Here's how the part is built. I have some questions about the finished solid (model axes, mm). Face numbers are marked on the shaded views. A direction names the side the tool comes from. Give positions to 0.01 mm unless a question says otherwise; leave off trailing zeros. Write each loop counter-clockwise with the first axis right and the second up, starting at its lowest first coordinate (ties: lowest second). Pieces come first, ordered by that corner, then holes. Notation, with made-up numbers: (-33, 26) - (-29, 26) arc R5 ccw to (-29, 31) - close; hole circle Ø7 at (19, -18.75). An arc over 180 degrees is marked (long way). One line per item, written item: value. Start each with the question number.
1) Imagine slicing it at C-C on y = 24.5. Write out the boundary of the cut face in (x, z).
2) Imagine slicing it at D-D on y = 66. Write out the boundary of the cut face in (x, z).
3) Imagine slicing it at A-A on x = -23. Write out the boundary of the cut face in (y, z), plus the area to 3 significant figures.
4) Imagine slicing it at B-B on z = 0. Write out the boundary of the cut face in (x, y) (3 decimals), plus the area to 3 significant figures.
5) We'd pull the mould along Y, two halves only. Please class the marked faces 1, 2, 3 and 4: +Y half, -Y half, draft (parallel to the pull), parting line (faces both ways), or undercut.
6) I'm going to push flat-ended pins straight in: P1, Ø6, axis at y = 13, z = 14.5, coming from the -X side; P2, Ø5, axis at x = -46.5, z = -15, coming from the -Y side; P3, Ø12, axis at y = 49, z = -1, coming from the -X side. Where does each tip first touch, or does it pass through?
7) On a 3-axis mill with a long thin cutter (end or side, diameter ignored), from which of +Z, -Z, +X, -X, +Y, -Y can I reach the whole of each face in a straight line? I mean the marked faces 5 and 6. Say none if no direction works.
8) Please list where these lines run through material, in increasing order: L1, parallel to Y at x = -27.5, z = 9; L2, parallel to X at y = 79, z = -14; L3, parallel to Y at x = -55.5, z = -8. Write a range as [from, to].
from build123d import *

# Parameters (mm, degrees)
EXTRUDE_THIN1_DEPTH = 19.05
SKETCH2_R           = 6.35
CUT_EXTRUDE1_DEPTH  = 10


with BuildPart() as part:
    # Sketch1 → Extrude-Thin1 (new, symmetric)
    with BuildSketch(Plane.XY):
        with BuildLine():
            Line((-77.216, 27.494), (-45.335245866, 0.74281114))
            ThreePointArc((-45.335245866, 0.74281114), (-44.380308124, 0.191476527), (-43.294392527, 0))
            Line((-43.294392527, 0), (-3.175, 0))
            ThreePointArc((-3.175, 0), (-0.92993597, 0.92993597), (0, 3.175))
            Line((0, 3.175), (0, 79.375))
            ThreePointArc((0, 79.375), (-0.92993597, 81.62006403), (-3.175, 82.55))
            Line((-3.175, 82.55), (-57.15, 82.55))
            Line((-57.15, 82.55), (-57.15, 88.9))
            Line((-57.15, 88.9), (-3.175, 88.9))
            ThreePointArc((-3.175, 88.9), (3.560192091, 86.110192091), (6.35, 79.375))
            Line((6.35, 79.375), (6.35, 3.175))
            ThreePointArc((6.35, 3.175), (3.560192091, -3.560192091), (-3.175, -6.35))
            Line((-3.175, -6.35), (-43.294392527, -6.35))
            ThreePointArc((-43.294392527, -6.35), (-46.55213932, -5.775570419), (-49.416952544, -4.121566579))
            Line((-49.416952544, -4.121566579), (-81.297706678, 22.629622281))
            Line((-81.297706678, 22.629622281), (-77.216, 27.494))
        make_face()
    extrude(amount=EXTRUDE_THIN1_DEPTH, both=True)

    # Sketch2 → Cut-Extrude1 (cut)
    with BuildSketch(Plane(origin=(0, 88.9, 0), x_dir=(1, 0, 0), z_dir=(0, 1, 0))):
        with Locations(Location((-44.45, 0, 0), (0, 0, 270))):
            Circle(SKETCH2_R)
    extrude(amount=-CUT_EXTRUDE1_DEPTH, mode=Mode.SUBTRACT)


solid = part.part
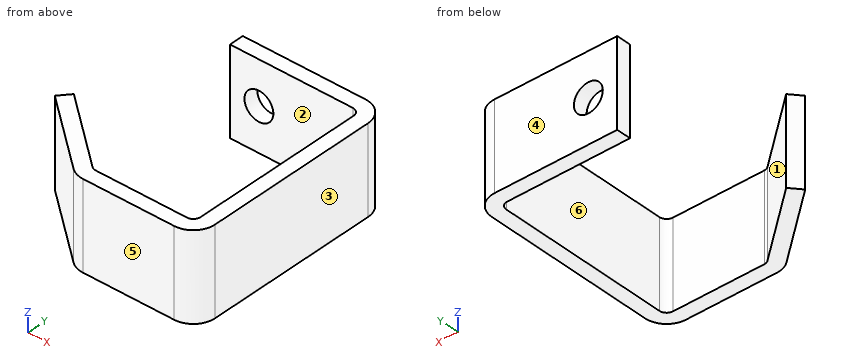
Numbers:
1. outline: (-79.73, -19.05) - (-73.65, -19.05) - (-73.65, 19.05) - (-79.73, 19.05) - close; (0, -19.05) - (6.35, -19.05) - (6.35, 19.05) - (0, 19.05) - close
2. outline: (0, -19.05) - (6.35, -19.05) - (6.35, 19.05) - (0, 19.05) - close
3. outline: (-6.35, -19.05) - (0, -19.05) - (0, 19.05) - (-6.35, 19.05) - close; (82.55, -19.05) - (88.9, -19.05) - (88.9, 19.05) - (82.55, 19.05) - close
3. area: 484 mm^2
4. outline: (-81.298, 22.63) - (-49.417, -4.122) arc R9.525 ccw to (-43.294, -6.35) - (-3.175, -6.35) arc R9.525 ccw to (6.35, 3.175) - (6.35, 79.375) arc R9.525 ccw to (-3.175, 88.9) - (-38.1, 88.9) - (-38.1, 82.55) - (-3.175, 82.55) arc R3.175 cw to (0, 79.375) - (0, 3.175) arc R3.175 cw to (-3.175, 0) - (-43.294, 0) arc R3.175 cw to (-45.335, 0.743) - (-77.216, 27.494) - close; (-57.15, 82.55) - (-50.8, 82.55) - (-50.8, 88.9) - (-57.15, 88.9) - close
4. area: 1,420 mm^2
5. face 1: undercut
5. face 2: undercut
5. face 3: draft
5. face 4: +Y half
6. P1: x = -73.4
6. P2: y = -6.32
6. P3: x = 0
7. face 5: +Z, -Z, +X, -X, -Y
7. face 6: +Z, -Z
8. L1: [-6.35, 0], [82.55, 88.9]
8. L2: [0, 6.35]
8. L3: [0.98, 9.27], [82.55, 88.9]
